from build123d import *

# Parameters (mm, degrees)
EXTRUDE_1_DEPTH     = 22
SKETCH_2_R          = 1.5
EXTRUDE_2_DEPTH     = 5
CHAMFER_1_SIZE      = 0.5
SKETCH_3_R          = 1.5
CUT_EXTRUDE_1_DEPTH = 10


with BuildPart() as part:
    # 草图1 → 凸台-拉伸1 (new body)
    with BuildSketch(Plane.XY):
        Polygon((3.175426481, 0), (1.58771324, 2.75), (-1.58771324, 2.75), (-3.175426481, 0), (-1.58771324, -2.75), (1.58771324, -2.75), align=None)
    extrude(amount=EXTRUDE_1_DEPTH)

    # 草图2 → 凸台-拉伸2 (add)
    with BuildSketch(Plane.XY.offset(22)):
        Circle(SKETCH_2_R)
    extrude(amount=EXTRUDE_2_DEPTH)

    # 倒角1
    chamfer_1_edges = [part.edges().sort_by_distance(p)[0] for p in [
        (-1.5, 0, 27),
    ]]
    chamfer(chamfer_1_edges, length=CHAMFER_1_SIZE)

    # 草图3 → 切除-拉伸1 (cut)
    with BuildSketch(Plane(origin=(0, 0, 0), x_dir=(-1, 0, 0), z_dir=(0, 0, -1))):
        Circle(SKETCH_3_R)
    extrude(amount=-CUT_EXTRUDE_1_DEPTH, mode=Mode.SUBTRACT)


solid = part.part
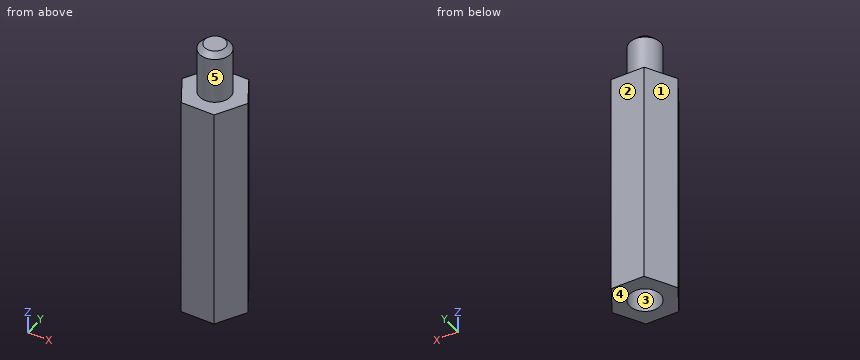
Source: CAD feature listing. Evaluate the final solid. Frame: model axes, mm. Face numbers are marked on the shaded views. A direction names the side the tool comes from. Round coordinates to 2 decimals unless told otherwise and drop trailing zeros. Loops run counter-clockwise (first coordinate to the right, second up) from the corner with the lowest first, then second, coordinate; pieces in that order, holes last.
Q1. Section A-A, the plane x = 0. Return loops of the section in (y, z).
Q2. Mould query, pull axis X, two halves, no side actions, for the marked faces 1, 2 and 3. Classes: pulls with the +X half, pulls with the -X half, needs draft (parallel to the pull), parting line crosses it, or undercut.
Q3. Ray query, line 1 (Y direction, x = 0, z = 6.75); line 2 (Z direction, x = -0.5, y = -1.65); line 3 (X direction, y = -0.35, z = 7.25). Return the intervals inside material, ascending.
Q4. Section B-B, the plane z = 6.5. Return loops of the section in (x, y).
Q5. First-contact query: P1, Ø1.5, axis at x = -0.5, y = 0, coming from the -Z side; P2, Ø3, axis at y = 0, z = 12, coming from the +X side. Flat tips, straight axial feed; report the tip coordinate or a pass-through.
Q6. Section D-D, the plane y = -2.1. Return loops of the section in (x, z), plus the area to 3 significant figures.
Q7. Section C-C, the plane z = 12. Return loops of the section in (x, y), plus the area to 3 significant figures.
Q8. Access query for the marked faces 4 and 5. Directions: +Z, -Z, +X, -X, +Y, -Y. A direction counts if a zero-diameter tool reaches every point of the face in a straight line with its end or side. Return the directions, or none.
Solutions:
1. outline: (-2.75, 0) - (-1.5, 0) - (-1.5, 10) - (1.5, 10) - (1.5, 0) - (2.75, 0) - (2.75, 22) - (1.5, 22) - (1.5, 26.5) - (1, 27) - (-1, 27) - (-1.5, 26.5) - (-1.5, 22) - (-2.75, 22) - close
2. face 1: pulls with the -X half
2. face 2: needs draft
2. face 3: undercut
3. line 1: y = -2.75 to -1.5, 1.5 to 2.75
3. line 2: z = 0 to 22
3. line 3: x = -2.97 to -1.46, 1.46 to 2.97
4. outline: (-3.18, 0) - (-1.59, -2.75) - (1.59, -2.75) - (3.18, 0) - (1.59, 2.75) - (-1.59, 2.75) - close; hole circle Ø3 at (0, 0)
5. P1: stops at z = 10
5. P2: stops at x = 3.18
6. outline: (-1.96, 0) - (1.96, 0) - (1.96, 22) - (-1.96, 22) - close
6. area: 86.4 mm2
7. outline: (-3.18, 0) - (-1.59, -2.75) - (1.59, -2.75) - (3.18, 0) - (1.59, 2.75) - (-1.59, 2.75) - close
7. area: 26.2 mm2
8. face 4: -Z, +X, -X, +Y, -Y
8. face 5: +Z
